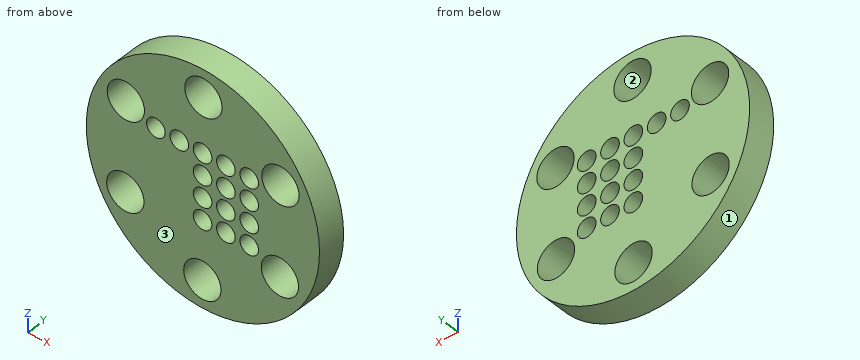
Autodesk Fusion 360 part; units mm, degrees
sketch "Sketch1" plane through (0, 0, 0) normal (0, 1, 0) x (1, 0, 0)
  circle A0 centre (0, 0) radius 125
extrude "Extrude1" add sketch "Sketch1" along normal blind 30
hole "Hole1" at (0.5541, 0, 95.6679) direction (0, 1, 0) diameter 40 depth 70 tip angle 118
pattern_circular "C-Pattern1" count 6 over 360 about axis through (0, 1.75, 0) along (0, 1, 0) of "Hole1"
hole "Hole2" at (-0.3403, 0, 37.0859) direction (0, 1, 0) diameter 20 depth 70 tip angle 118
pattern_linear "R-Pattern1" count 3 spacing 25 along (1, 0, 0) count 4 spacing 23.3333 along (0, 0, -1) of "Hole2"
pattern_linear "R-Pattern2" count 3 spacing 25 along (-1, 0, 0) of "Hole2"
Build history of the part. All positions in model axes, mm. Face numbers are marked on the shaded views. Round coordinates to 2 decimals unless told otherwise and drop trailing zeros. Write each loop counter-clockwise with the first axis right and the second up, starting at its lowest first coordinate (ties: lowest second). Pieces come first, ordered by that corner, then holes.
1) Band-saw the part on C-C, the plane x = -75. List the corners of the cut face in (y, z), and give its area (3 significant figures).
2) Band-saw the part on D-D, the plane x = -5. List the corners of the cut face in (y, z), and give its area (3 significant figures).
3) Band-saw the part on A-A, the plane z = -52.5. List the corners of the cut face in (x, y).
4) Mould opens along X. For the marked faces 1, 2 and 3 say: +X half, -X half, draft (parallel to the pull), parting line (faces both ways), or undercut.
5) Pin check, flat tips, straight feed: pin 1 (4 mm diameter, centred on x = 14.5, y = 6.5, fed in from -Z); pin 2 (18 mm diameter, centred on x = 24.66, z = 37.09, fed in from -Y); pin 3 (3 mm diameter, centred on y = 9.5, z = -51, fed in from -X); pin 4 (3 mm diameter, centred on y = 25.5, z = -45, fed in from +X). Stop position of each tip, or through.
6) Band-saw the part on B-B, the plane y = 24.5. Give the number of separate pieces and of enclosed holes in the cut face, and give its area (3 significant figures).
7) Drill centre lines: probe 1 along X at (y, z) = (26.75, -18); probe 2 along Z at (x, y) = (85.5, 25); probe 3 along Z at (x, y) = (33.5, 2) (3 decimals). Where is each one in solid material? Low to high.
Ans:
1. outline: (0, -100) - (30, -100) - (30, -65.63) - (0, -65.63) - close; (0, -29.08) - (30, -29.08) - (30, 29.8) - (0, 29.8) - close; (0, 66.82) - (30, 66.82) - (30, 100) - (0, 100) - close
1. area: 3,790 mm2
2. outline: (0, -124.9) - (30, -124.9) - (30, -115.17) - (0, -115.17) - close; (0, -76.17) - (30, -76.17) - (30, -41.76) - (0, -41.76) - close; (0, -24.07) - (30, -24.07) - (30, -18.43) - (0, -18.43) - close; (0, -0.73) - (30, -0.73) - (30, 4.9) - (0, 4.9) - close; (0, 22.6) - (30, 22.6) - (30, 28.24) - (0, 28.24) - close; (0, 45.93) - (30, 45.93) - (30, 76.45) - (0, 76.45) - close; (0, 114.88) - (30, 114.88) - (30, 124.9) - (0, 124.9) - close
2. area: 3,050 mm2
3. outline: (-113.44, 0) - (-102.45, 0) - (-102.45, 30) - (-113.44, 30) - close; (-63.8, 0) - (63.02, 0) - (63.02, 30) - (-63.8, 30) - close; (102.13, 0) - (113.44, 0) - (113.44, 30) - (102.13, 30) - close
4. face 1: parting line
4. face 2: undercut
4. face 3: draft
5. pin 1: stops at z = -124.37
5. pin 2: passes through
5. pin 3: stops at x = -114.78
5. pin 4: stops at x = 117.19
6. separate pieces: 1
6. enclosed holes: 20
6. area: 37,100 mm2
7. probe 1: x = -123.7 to -5.74, 5.06 to 19.26, 30.06 to 44.26, 55.06 to 123.7
7. probe 2: z = -91.19 to -68.1, -28.53 to 27.5, 67.21 to 91.19
7. probe 3: z = -120.427 to -37.588, -28.24 to -14.255, -4.906 to 9.078, 18.427 to 32.412, 41.76 to 120.427
